For this review, take the finished solid that the model builds, in its own axes (mm). A direction names the side the tool comes from. Round coordinates to 2 decimals unless told otherwise and drop trailing zeros. Order: outer loops, then holes, each group sorted by start corner. A loop starts at its lowest first (then second) coordinate and runs counter-clockwise, first axis right, second up.
```python
from build123d import *

# Parameters (mm, degrees)
SKETCH2_R                      = 6
CUT_EXTRUDE1_DEPTH             = 201
CIRPATTERN1_COUNT              = 4
SKETCH3_R                      = 24
CUT_EXTRUDE2_DEPTH             = 144
BOSS_EXTRUDE2_DEPTH            = 20
CUT_EXTRUDE3_REACH             = 222
SKETCH8_R                      = 6
CUT_EXTRUDE4_REACH             = 222
SKETCH10_R                     = 5.551973051
CUT_EXTRUDE5_REACH             = 222
SKETCH11_R                     = 5
CUT_EXTRUDE6_REACH             = 222
SKETCH12_R                     = 5
CUT_EXTRUDE6_DIRECTION_2_DEPTH = 1


with BuildPart() as part:
    # Sketch1 → Revolve1 (revolve)
    with BuildSketch(Plane.XY):
        Polygon((0, 0), (15, 0), (15, 50), (30, 50), (30, 180), (60, 180), (60, 200), (0, 200), align=None)
    revolve(axis=Axis((0, 218.08318264, 0), (0, -1, 0)))

    # Sketch2 → Cut-Extrude1 (cut, through all)
    with BuildSketch(Plane(origin=(0, 200, 0), x_dir=(1, 0, 0), z_dir=(0, 1, 0))):
        with Locations((0, 45)):
            Circle(SKETCH2_R)
    cut_extrude1 = extrude(amount=-CUT_EXTRUDE1_DEPTH, mode=Mode.SUBTRACT)

    # CirPattern1: Cut-Extrude1 ×4 about axis
    cirpattern1_axis = Axis((0, 0, 0), (0, 1, 0))
    for i in range(1, CIRPATTERN1_COUNT):
        add(cut_extrude1.rotate(cirpattern1_axis, i * 360 / CIRPATTERN1_COUNT), mode=Mode.SUBTRACT)

    # Sketch3 → Cut-Extrude2 (cut)
    with BuildSketch(Plane(origin=(0, 200, 0), x_dir=(1, 0, 0), z_dir=(0, 1, 0))):
        Circle(SKETCH3_R)
    extrude(amount=-CUT_EXTRUDE2_DEPTH, mode=Mode.SUBTRACT)

    # Sketch4 → Boss-Extrude2 (add)
    with BuildSketch(Plane.XZ):
        with BuildLine():
            Line((-25, 35), (25, 35))
            ThreePointArc((25, 35), (32.071067812, 32.071067812), (35, 25))
            Line((35, 25), (35, -25))
            ThreePointArc((35, -25), (32.071067812, -32.071067812), (25, -35))
            Line((25, -35), (-25, -35))
            ThreePointArc((-25, -35), (-32.071067812, -32.071067812), (-35, -25))
            Line((-35, -25), (-35, 25))
            ThreePointArc((-35, 25), (-32.071067812, 32.071067812), (-25, 35))
        make_face()
    extrude(amount=BOSS_EXTRUDE2_DEPTH)

    # Sketch8 → Cut-Extrude3 (cut, up to next)
    with BuildSketch(Plane.XZ.offset(20), mode=Mode.PRIVATE) as cut_extrude3_sk1:
        with Locations((-25, 25)):
            Circle(SKETCH8_R)
    cut_extrude3_tool1 = extrude(cut_extrude3_sk1.sketch, amount=-CUT_EXTRUDE3_REACH, mode=Mode.PRIVATE) & part.part
    add(cut_extrude3_tool1.solids().sort_by_distance((-25, -20, 25))[0], mode=Mode.SUBTRACT)

    # Sketch10 → Cut-Extrude4 (cut, up to next)
    with BuildSketch(Plane(origin=(0, -20, 0), x_dir=(-1, 0, 0), z_dir=(0, -1, 0)), mode=Mode.PRIVATE) as cut_extrude4_sk1:
        with Locations((-25, -25)):
            Circle(SKETCH10_R)
    cut_extrude4_tool1 = extrude(cut_extrude4_sk1.sketch, amount=-CUT_EXTRUDE4_REACH, mode=Mode.PRIVATE) & part.part
    add(cut_extrude4_tool1.solids().sort_by_distance((25, -20, 25))[0], mode=Mode.SUBTRACT)

    # Sketch11 → Cut-Extrude5 (cut, up to next)
    with BuildSketch(Plane(origin=(0, -20, 0), x_dir=(-1, 0, 0), z_dir=(0, -1, 0)), mode=Mode.PRIVATE) as cut_extrude5_sk1:
        with Locations((-25, 25)):
            Circle(SKETCH11_R)
    cut_extrude5_tool1 = extrude(cut_extrude5_sk1.sketch, amount=-CUT_EXTRUDE5_REACH, mode=Mode.PRIVATE) & part.part
    add(cut_extrude5_tool1.solids().sort_by_distance((25, -20, -25))[0], mode=Mode.SUBTRACT)

    # Sketch12 → Cut-Extrude6 (cut, up to next)
    with BuildSketch(Plane.XZ.offset(20), mode=Mode.PRIVATE) as cut_extrude6_sk1:
        with Locations((-25, -25)):
            Circle(SKETCH12_R)
    cut_extrude6_tool1 = extrude(cut_extrude6_sk1.sketch, amount=-CUT_EXTRUDE6_REACH, mode=Mode.PRIVATE) & part.part
    add(cut_extrude6_tool1.solids().sort_by_distance((-25, -20, -25))[0], mode=Mode.SUBTRACT)

    # Sketch12 → Cut-Extrude6 direction 2 (cut)
    with BuildSketch(Plane.XZ.offset(20)):
        with Locations((-25, -25)):
            Circle(SKETCH12_R)
    extrude(amount=CUT_EXTRUDE6_DIRECTION_2_DEPTH, mode=Mode.SUBTRACT)


solid = part.part
```
Q1. Take a section at D-D, the plane z = 45. State the section outline as (x, y) points.
Q2. Take a section at A-A, the plane z = 0. State the section outline as (x, y) points, plus the area to 3 significant figures.
Q3. Take a section at C-C, the plane y = 172. State the section outline as (x, z) points, plus the area to 3 significant figures.
Q4. Take a section at B-B, the plane x = 0. State the section outline as (y, z) points, plus the area to 3 significant figures.
Q5. Clearance check with flat-ended pins moving along their axes: pin 1 (16 mm diameter, centred on y = -14.5, z = -5, fed in from -X); pin 2 (10 mm diameter, centred on y = -12.5, z = -6.5, fed in from +X); pin 3 (10 mm diameter, centred on x = 11.5, y = -5.5, fed in from -Z). State where each tip first meets the part, or that it passes through.
Q6. Mouldability with a two-part tool opening along Y and no side actions: class faces 4 (the face through (-29.97, 115.91, 1.32)), 5 (the face through (-14.985, 25.35, 0.66)), 6 (the face through (-32.15, -9.86, 31.99)), 7 (the face through (26, 200, 1)) as +Y half, -Y half, draft (parallel to the pull), parting line (faces both ways), or undercut.
Q7. Wall thickness on line 1 (Z direction, x = 25, y = -6.25); line 2 (Y direction, x = -13, z = 11.5); line 3 (Y direction, x = 8, z = -24.5): over which ranges is each line inside the solid? List them lowest first.
Q8. Tool access review of faces 1 (the face through (0, -10, 35)), 2 (the face through (30.547, -10.14, 24.756)), 3 (the face through (-31.99, -9.86, -32.15)): name each direction out of +Z, -Z, +X, -X, +Y, -Y from which nothing blocks a thin tool from reaching the whole face with its end or side.
Working result:
1. outline: (-39.69, 180) - (-6, 180) - (-6, 200) - (-39.69, 200) - close; (6, 180) - (39.69, 180) - (39.69, 200) - (6, 200) - close
2. outline: (-60, 180) - (-51, 180) - (-51, 200) - (-60, 200) - close; (-39, 180) - (-30, 180) - (-30, 50) - (-15, 50) - (-15, 0) - (-35, 0) - (-35, -20) - (35, -20) - (35, 0) - (15, 0) - (15, 50) - (30, 50) - (30, 180) - (39, 180) - (39, 200) - (24, 200) - (24, 56) - (-24, 56) - (-24, 200) - (-39, 200) - close; (51, 180) - (60, 180) - (60, 200) - (51, 200) - close
2. area: 5,710 mm2
3. outline: circle Ø60 at (0, 0); hole circle Ø48 at (0, 0)
3. area: 1,020 mm2
4. outline: (-20, -35) - (0, -35) - (0, -15) - (50, -15) - (50, -30) - (180, -30) - (180, -39) - (200, -39) - (200, -24) - (56, -24) - (56, 24) - (200, 24) - (200, 39) - (180, 39) - (180, 30) - (50, 30) - (50, 15) - (0, 15) - (0, 35) - (-20, 35) - close; (180, -60) - (200, -60) - (200, -51) - (180, -51) - close; (180, 51) - (200, 51) - (200, 60) - (180, 60) - close
4. area: 5,710 mm2
5. pin 1: stops at x = -35
5. pin 2: stops at x = 35
5. pin 3: stops at z = -35
6. face 4: undercut
6. face 5: undercut
6. face 6: draft
6. face 7: +Y half
7. line 1: z = -35 to -30, -20 to 19.45, 30.55 to 35
7. line 2: y = -20 to 0, 50 to 56
7. line 3: y = -20 to 0, 50 to 200
8. face 1: +Z, +X, -X, -Y
8. face 2: -Y
8. face 3: -Z, -X, -Y
